Geometry: see drawing. Coordinates: mm, zero at the bounding-box minimum. Round coordinates to 2 decimals unless told otherwise and drop trailing zeros. Write each loop counter-clockwise with the first axis right and the second up, starting at its lowest first coordinate (ties: lowest second). Pieces come first, ordered by that corner, then holes. Notation, with made-up numbers: (68.5, 46.25) -> (75.5, 46.25) arc R17 ccw to (75.5, 55.25) -> close; hole circle Ø6 at (9.25, 0.5). An arc over 180 degrees is marked (long way). Write item = value, one per line.
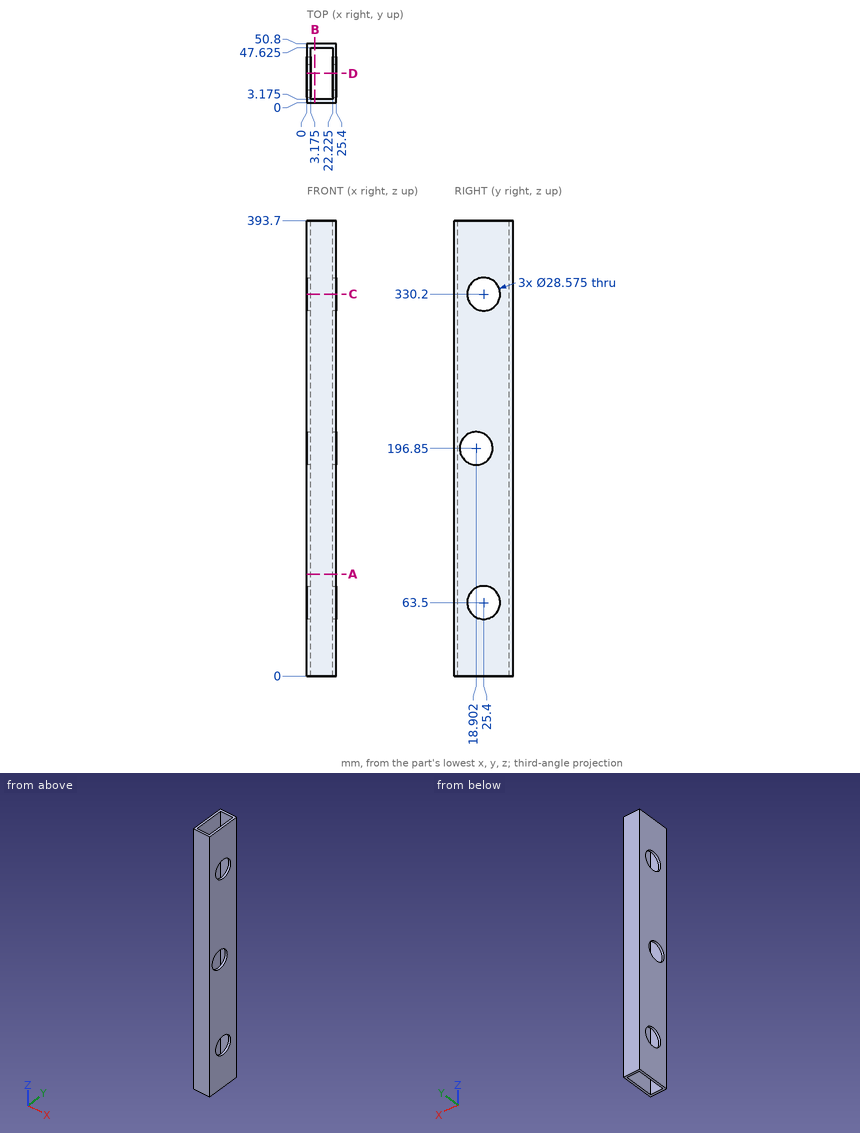
1) Cut plane A-A (z = 88). Return the cut outline in (x, y) (1 decimal).
Solutions:
outline = (0, 0) -> (25.4, 0) -> (25.4, 50.8) -> (0, 50.8) -> close; hole (3.2, 3.2) -> (22.2, 3.2) -> (22.2, 47.6) -> (3.2, 47.6) -> close
2) Cut plane C-C (z = 330.2). Return the cut outline in (x, y) (1 decimal).
Solutions:
outline = (0, 0) -> (25.4, 0) -> (25.4, 11.1) -> (22.2, 11.1) -> (22.2, 3.2) -> (3.2, 3.2) -> (3.2, 11.1) -> (0, 11.1) -> close; (0, 39.7) -> (3.2, 39.7) -> (3.2, 47.6) -> (22.2, 47.6) -> (22.2, 39.7) -> (25.4, 39.7) -> (25.4, 50.8) -> (0, 50.8) -> close
3) Cut plane D-D (y = 25.4). Count the separate pieces of the cut face and the enclosed holes in it.
Solutions:
separate_pieces = 8
enclosed_holes = 0
4) First-contact query: P1, Ø5, axis at x = 3.5, z = 143.5, coming from the -Y side; P2, Ø3, axis at x = 5.5, y = 23.5, coming from the -Z side. Flat tips, straight axial feed; report the tip coordinate or a pass-through.
Solutions:
P1 = 0
P2 = through
5) Line query: L1, parallel to X at y = 36.5, z = 37 (1 decimal); L2, parallel to Y at x = 18, z = 305 (1 decimal); L3, parallel to Y at x = 23.9, z = 196.85. Output: solid intervals per line, ascending. Write a range as from..to.
Solutions:
L1 = 0..3.2, 22.2..25.4
L2 = 0..3.2, 47.6..50.8
L3 = 0..4.61, 33.19..50.8
6) Cut plane B-B (x = 6.75). Return the cut outline in (y, z) (1 decimal), and give its area (3 significant figures).
Solutions:
outline = (0, 0) -> (3.2, 0) -> (3.2, 393.7) -> (0, 393.7) -> close; (47.6, 0) -> (50.8, 0) -> (50.8, 393.7) -> (47.6, 393.7) -> close
area = 2,500 mm^2
